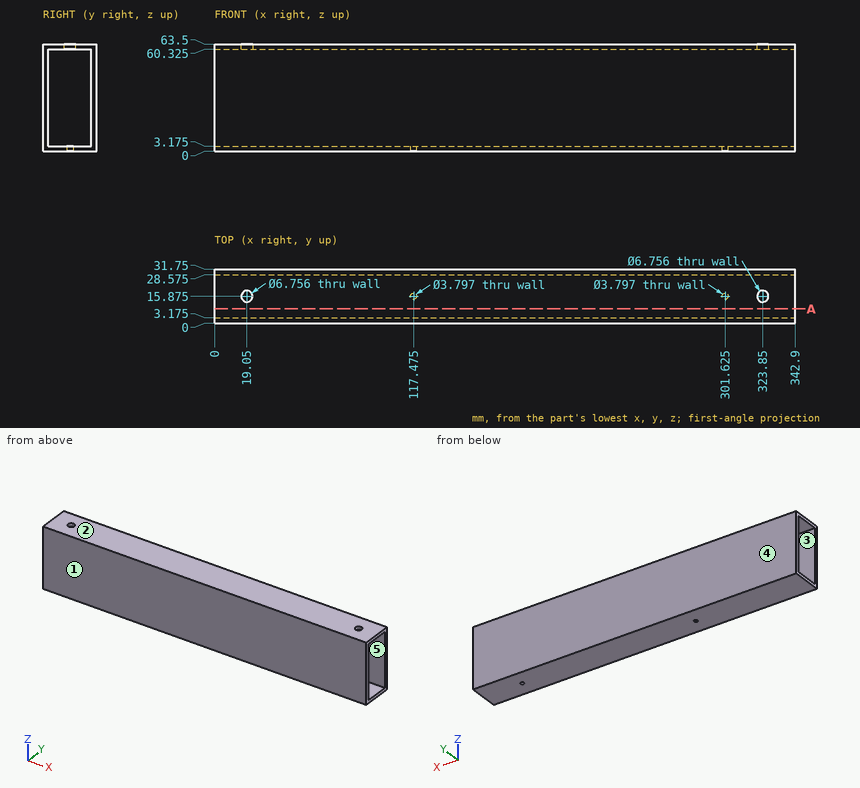
Check sheet for the drawn part. Datum: minimum x, y, z corner. Units: mm. A direction names the side the tool comes from. Round coordinates to 2 decimals unless told otherwise and drop trailing zeros. Order: outer loops, then holes, each group sorted by start corner. A loop starts at its lowest first (then second) coordinate and runs counter-clockwise, first axis right, second up. Notation, with made-up numbers: M 18,30 L 65,30 A14 cw 65,52 Z; hole C 2,65 d11. An arc over 180 degrees is marked long. Answer in a Markdown table with one row per item.
(1) Set-up check for the marked faces 4 and 5: record each of +Z, -Z, +X, -X, +Y, -Y from which the full face is reachable in a straight line by a thin tool's end or side.
Findings:
| item | result |
|---|---|
| face 4 | +Z, -Z, +X, -X, +Y |
| face 5 | +X, -X |
(2) Section check A-A on y = 8.5. Record the boundary of the cut face in (x, z) (1 decimal).
Findings:
| item | result |
|---|---|
| outline | M 0,0 L 342.9,0 L 342.9,3.2 L 0,3.2 Z; M 0,60.3 L 342.9,60.3 L 342.9,63.5 L 0,63.5 Z |
(3) Gauge pin test, flat ends, axial feed: pin 1 (1 mm diameter, centred on x = 223, z = 17.5, fed in from -Y); pin 2 (3.5 mm diameter, centred on x = 301.625, y = 15.875, fed in from -Z) (3 decimals). Record the tip position at first contact, or that the pin passes through.
Findings:
| item | result |
|---|---|
| pin 1 | stops at y = 0 |
| pin 2 | stops at z = 60.325 |
(4) Material ranges on line 1 along Z through (x, y) = (94, 18) (1 decimal); line 2 along Y through (x, z) = (19.05, 62.4); line 3 along Z through (x, y) = (117, 15.5) (1 decimal), recorded low to high. Write a range as from..to.
Findings:
| item | result |
|---|---|
| line 1 | z = 0..3.2, 60.3..63.5 |
| line 2 | y = 0..12.5, 19.25..31.75 |
| line 3 | z = 60.3..63.5 |
(5) Draft check along Y on the marked faces 1, 2 and 3. Enter one of: +Y half, -Y half, draft (parallel to the pull), parting line (faces both ways), or undercut.
Findings:
| item | result |
|---|---|
| face 1 | -Y half |
| face 2 | draft |
| face 3 | undercut |
